Part model, mm, in its own coordinate system. Give positions to 0.01 mm unless a question says otherwise; leave off trailing zeros. Order: outer loops, then holes, each group sorted by start corner. A loop starts at its lowest first (then second) coordinate and runs counter-clockwise, first axis right, second up. Notation, with made-up numbers: M -11.75,-22 L -1.75,-22 A20 ccw -1.75,4 Z; hole C -2.75,86 d10. An arc over 180 degrees is marked long. Return JSON: item names as keys, results as strings.
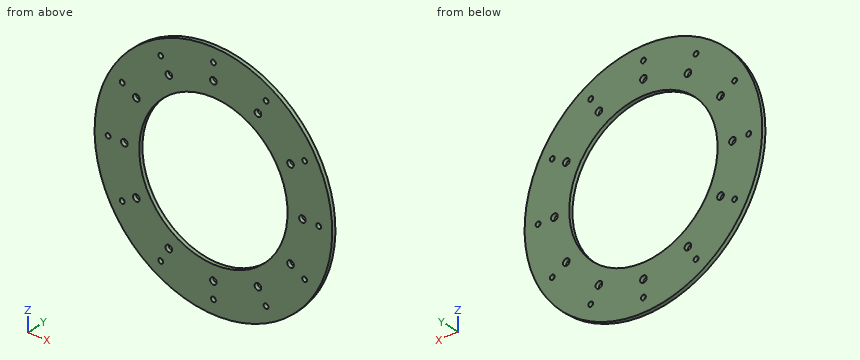
from build123d import *

# Parameters (mm, degrees)
SKETCH1_R           = 79
SKETCH1_R_2         = 49.3
BOSS_EXTRUDE1_DEPTH = 2.5
SKETCH2_R           = 1.6
CUT_EXTRUDE1_DEPTH  = 112.750838923
SKETCH3_R           = 2.2
CUT_EXTRUDE2_DEPTH  = 112.750838923


with BuildPart() as part:
    # Sketch1 → Boss-Extrude1 (new body)
    with BuildSketch(Plane(origin=(0, 0, 0), x_dir=(1, 0, 0), z_dir=(0, 1, 0))):
        with Locations(Location((0, 0, 0), (0, 0, 270))):
            Circle(SKETCH1_R)
        with Locations(Location((0, 0, 0), (0, 0, 270))):
            Circle(SKETCH1_R_2, mode=Mode.SUBTRACT)
    extrude(amount=BOSS_EXTRUDE1_DEPTH)

    # Sketch2 → Cut-Extrude1 (cut, through all)
    with BuildSketch(Plane(origin=(0, 2.5, 0), x_dir=(1, 0, 0), z_dir=(0, 1, 0))):
        with Locations(Location((0, 70, 0), (0, 0, 270))):
            Circle(SKETCH2_R)
        with Locations(Location((35, 60.621778265, 0), (0, 0, 270))):
            Circle(SKETCH2_R)
        with Locations(Location((60.621778265, 35, 0), (0, 0, 270))):
            Circle(SKETCH2_R)
        with Locations(Location((70, 0, 0), (0, 0, 270))):
            Circle(SKETCH2_R)
        with Locations(Location((60.621778265, -35, 0), (0, 0, 270))):
            Circle(SKETCH2_R)
        with Locations(Location((35, -60.621778265, 0), (0, 0, 270))):
            Circle(SKETCH2_R)
        with Locations(Location((0, -70, 0), (0, 0, 270))):
            Circle(SKETCH2_R)
        with Locations(Location((-35, -60.621778265, 0), (0, 0, 270))):
            Circle(SKETCH2_R)
        with Locations(Location((-60.621778265, -35, 0), (0, 0, 270))):
            Circle(SKETCH2_R)
        with Locations(Location((-70, 0, 0), (0, 0, 270))):
            Circle(SKETCH2_R)
        with Locations(Location((-60.621778265, 35, 0), (0, 0, 270))):
            Circle(SKETCH2_R)
        with Locations(Location((-35, 60.621778265, 0), (0, 0, 270))):
            Circle(SKETCH2_R)
    extrude(amount=-CUT_EXTRUDE1_DEPTH, mode=Mode.SUBTRACT)

    # Sketch3 → Cut-Extrude2 (cut, through all)
    with BuildSketch(Plane(origin=(0, 2.5, 0), x_dir=(1, 0, 0), z_dir=(0, 1, 0))):
        with Locations(Location((0, 59.18, 0), (0, 0, 270))):
            Circle(SKETCH3_R)
        with Locations(Location((29.59, 51.251383396, 0), (0, 0, 270))):
            Circle(SKETCH3_R)
        with Locations(Location((51.251383396, 29.59, 0), (0, 0, 270))):
            Circle(SKETCH3_R)
        with Locations(Location((59.18, 0, 0), (0, 0, 270))):
            Circle(SKETCH3_R)
        with Locations(Location((51.251383396, -29.59, 0), (0, 0, 270))):
            Circle(SKETCH3_R)
        with Locations(Location((29.59, -51.251383396, 0), (0, 0, 270))):
            Circle(SKETCH3_R)
        with Locations(Location((0, -59.18, 0), (0, 0, 270))):
            Circle(SKETCH3_R)
        with Locations(Location((-29.59, -51.251383396, 0), (0, 0, 270))):
            Circle(SKETCH3_R)
        with Locations(Location((-51.251383396, -29.59, 0), (0, 0, 270))):
            Circle(SKETCH3_R)
        with Locations(Location((-59.18, 0, 0), (0, 0, 270))):
            Circle(SKETCH3_R)
        with Locations(Location((-51.251383396, 29.59, 0), (0, 0, 270))):
            Circle(SKETCH3_R)
        with Locations(Location((-29.59, 51.251383396, 0), (0, 0, 270))):
            Circle(SKETCH3_R)
    extrude(amount=-CUT_EXTRUDE2_DEPTH, mode=Mode.SUBTRACT)


solid = part.part
Q1. Band-saw the part on C-C (y = 1.8). Give the number of separate pieces and of enclosed holes in the cut face, then the cut area to 3 significant figures.
Established:
{"separate pieces": "1", "enclosed holes": "25", "area": "11,700 mm²"}
Q2. Band-saw the part on A-A (x = 10). Give the cut face in (y, z), then the cut area to 3 significant figures.
Established:
{"outline": "M 0,-78.36 L 2.5,-78.36 L 2.5,-48.28 L 0,-48.28 Z; M 0,48.28 L 2.5,48.28 L 2.5,78.36 L 0,78.36 Z", "area": "150 mm²"}
Q3. Probe line 1 along X through (y, z) = (1.3, 0); line 2 along Z through (x, y) = (62, 0.3); line 3 along X through (y, z) = (1.85, 35). List the from-to ranges inside material, lowest first.
Established:
{"line 1": "x = -79 to -71.6, -68.4 to -61.38, -56.98 to -49.3, 49.3 to 56.98, 61.38 to 68.4, 71.6 to 79", "line 2": "z = -48.96 to -35.81, -34.19 to 34.19, 35.81 to 48.96", "line 3": "x = -70.82 to -62.22, -59.02 to -34.72, 34.72 to 59.02, 62.22 to 70.82"}
Q4. Pin check, flat tips, straight feed: pin 1 (5 mm diameter, centred on x = -16.5, z = 59, fed in from -Y); pin 2 (4 mm diameter, centred on x = -29.59, z = -51.25, fed in from +Y); pin 3 (1 mm diameter, centred on x = -58.5, y = 2, fed in from +Z). Stop position of each tip, or through.
Established:
{"pin 1": "stops at y = 0", "pin 2": "passes through", "pin 3": "stops at z = 53.64"}
Q5. Band-saw the part on D-D (x = -29.59). Give the cut face in (y, z).
Established:
{"outline": "M 0,-73.25 L 2.5,-73.25 L 2.5,-53.45 L 0,-53.45 Z; M 0,-49.05 L 2.5,-49.05 L 2.5,-39.43 L 0,-39.43 Z; M 0,39.43 L 2.5,39.43 L 2.5,49.05 L 0,49.05 Z; M 0,53.45 L 2.5,53.45 L 2.5,73.25 L 0,73.25 Z"}
Q6. Band-saw the part on B-B (z = 10.5). Give the cut face in (x, y).
Established:
{"outline": "M -78.3,0 L -48.17,0 L -48.17,2.5 L -78.3,2.5 Z; M 48.17,0 L 78.3,0 L 78.3,2.5 L 48.17,2.5 Z"}
